Job drawing, mm, ordinate dimensions from the low corner. One solid piece. A direction names the side the tool comes from. Round coordinates to 2 decimals unless told otherwise and drop trailing zeros. Loops run counter-clockwise (first coordinate to the right, second up) from the corner with the lowest first, then second, coordinate; pieces in that order, holes last. Notation, with made-up numbers: M 79,85.5 L 122,85.5 A18 ccw 122,89.5 Z; hole C 54.25,38.25 d5. An arc over 180 degrees is marked long. Put each result on its own line as item: value. Start each with the question number.
1) Which spindle directions (+Z, -Z, +X, -X, +Y, -Y) get a long thin tool onto all of the face, cutting with end or side? Do the marked faces 4, 5, 6, 7 and 8. Say none if no direction does.
2) Slice it at B-B on z = 7.25. Give the cut face in (x, y), then the cut area to 3 significant figures.
3) Slice it at D-D on z = 5.5. Give the cut face in (x, y).
4) Drop flat-ended pins along their axis: pin 1 Ø4 at (x, z) = (25.5, 4) entering from +Y; pin 2 Ø4 at (y, z) = (5, 4) entering from +X; pin 3 Ø1.8 at (y, z) = (17.5, 3) entering from -X. Give the stop position or say it passes through.
5) Slice it at A-A on x = 12.05. Give the cut face in (y, z).
6) Pull direction X, two halves, no side cores. Call the marked faces 1, 2 and 3: +X half, -X half, draft (parallel to the pull), parting line (faces both ways), or undercut.
7) Probe line 1 along Y through (x, z) = (2.75, 7.5); line 2 along X through (y, z) = (3, 1.75); line 3 along Y through (x, z) = (13.75, 2.25). List the from-to ranges inside material, lowest first.
8) Slice it at C-C on y = 5.75. Give the cut face in (x, z), then the cut area to 3 significant figures.
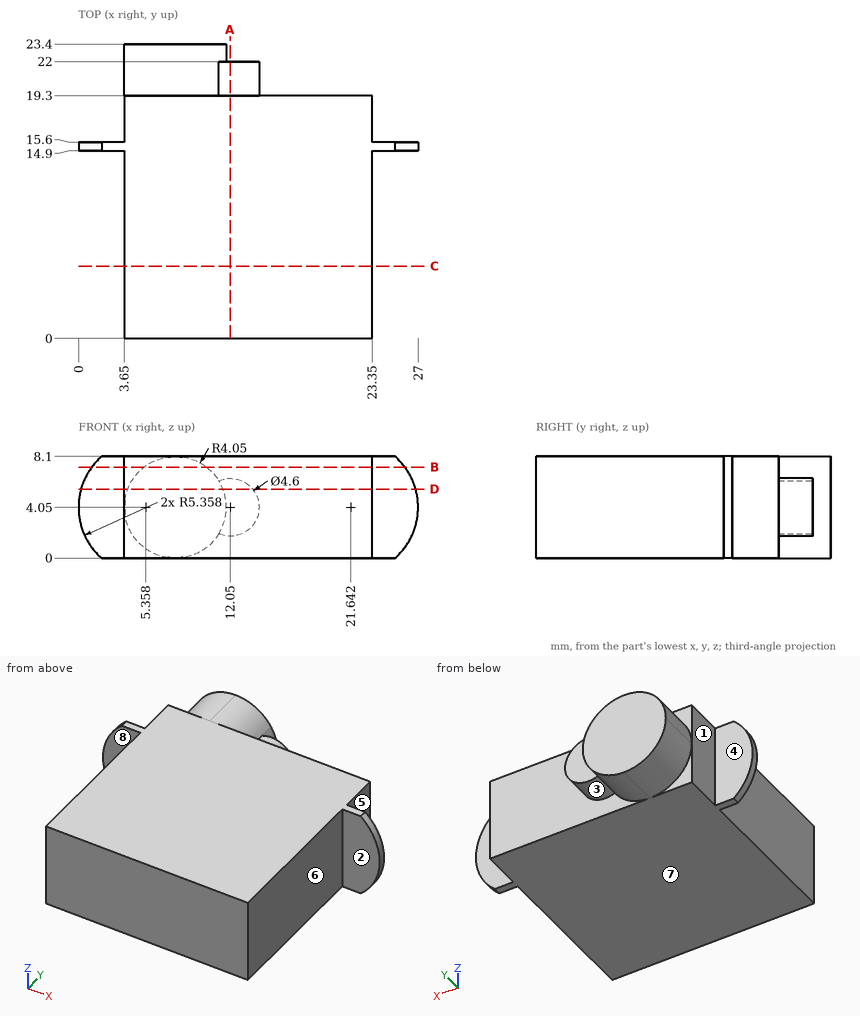
Recorded:
1. face 4: +Z, -Z, -X, +Y
1. face 5: +Z, -Z, +X, +Y
1. face 6: +Z, -Z, +X, -Y
1. face 7: -Z, +X, -X, +Y, -Y
1. face 8: +Z, -Z, -X, -Y
2. outline: M 1.06,14.9 L 3.65,14.9 L 3.65,0 L 23.35,0 L 23.35,14.9 L 25.94,14.9 L 25.94,15.6 L 23.35,15.6 L 23.35,19.3 L 10.18,19.3 L 10.18,23.4 L 5.22,23.4 L 5.22,19.3 L 3.65,19.3 L 3.65,15.6 L 1.06,15.6 Z
2. area: 404 mm2
3. outline: M 0.2,14.9 L 3.65,14.9 L 3.65,0 L 23.35,0 L 23.35,14.9 L 26.8,14.9 L 26.8,15.6 L 23.35,15.6 L 23.35,19.3 L 13.84,19.3 L 13.84,22 L 11.48,22 L 11.48,23.4 L 3.92,23.4 L 3.92,19.3 L 3.65,19.3 L 3.65,15.6 L 0.2,15.6 Z
4. pin 1: stops at y = 15.6
4. pin 2: stops at x = 23.35
4. pin 3: stops at x = 3.65
5. outline: M 0,0 L 19.3,0 L 19.3,1.75 L 22,1.75 L 22,6.35 L 19.3,6.35 L 19.3,8.1 L 0,8.1 Z
6. face 1: -X half
6. face 2: draft
6. face 3: undercut
7. line 1: y = 14.9 to 15.6
7. line 2: x = 3.65 to 23.35
7. line 3: y = 0 to 19.3
8. outline: M 3.65,0 L 23.35,0 L 23.35,8.1 L 3.65,8.1 Z
8. area: 160 mm2
